Can you work these out from the model? Positions are in its coordinate system, mm. A direction names the side the tool comes from. Round coordinates to 2 decimals unless told otherwise and drop trailing zeros. Loops run counter-clockwise (first coordinate to the right, second up) from the corner with the lowest first, then second, coordinate; pieces in that order, holes last.
(1) Will these pins go through, and if not, where does the flat tip stop? pin 1 Ø3.5 at (x, z) = (-17, 1) entering from +Y; pin 2 Ø1 at (x, z) = (4, 1) entering from +Y; pin 3 Ø1.2 at (y, z) = (-2, 1) entering from +X; pin 4 Ø10 at (x, y) = (-12.5, 6.5) entering from -Z.
(2) I want a section at D-D on y = 21.5. Write out the boundary of the cut face in (x, z), plus the area to 3 significant figures.
(3) I want a section at B-B on z = -1. Write out the boundary of the cut face in (x, y), plus the area to 3 significant figures.
(4) If I drill on line 1 along X through (y, z) = (12, 0.25); line 2 along X through (y, z) = (-5.5, 2.75); line 3 along Y through (x, z) = (30, 3.5), over which ranges is the centre line in solid material (lowest first)?
(5) I want a section at C-C on y = 0.5. Write out the boundary of the cut face in (x, z).
(6) Thinking about a two-plate mould opening in Y: for faces 1 (the face through (-44, 0, -1)), 2 (the face through (0, -21.5, -1)), 3 (the face through (1, -30, -1)), which applies, released by +Y, released by -Y, zero draft, split by the parting line, or undercut?
(7) I want a section at A-A on x = 23. Write out the boundary of the cut face in (y, z).
(8) Which directions (+Z, -Z, +X, -X, +Y, -Y) give clear straight access to the entire face, cutting with the end or side of a thin tool? Please do faces 4 (the face through (20, -12.5, 1)), 5 (the face through (-1, -22.5, 2)), 6 (the face through (14, 16, 1)).
from build123d import *

# Parameters (mm, degrees)
SKETCH5_W           = 85
SKETCH5_H           = 45
SKETCH5_W_2         = 72
SKETCH5_H_2         = 25
BOSS_EXTRUDE3_DEPTH = 4
SKETCH10_W          = 88
SKETCH10_H          = 60
SKETCH10_W_2        = 72
SKETCH10_H_2        = 25
BOSS_EXTRUDE4_DEPTH = 3
SKETCH12_W          = 4
SKETCH12_H          = 15
CUT_EXTRUDE6_DEPTH  = 3
SKETCH13_W          = 43
SKETCH13_H          = 6
CUT_EXTRUDE7_DEPTH  = 3
SKETCH18_W          = 6.2
SKETCH18_H          = 5
CUT_EXTRUDE10_DEPTH = 9
SKETCH19_W          = 6.2
SKETCH19_H          = 0.5
CUT_EXTRUDE11_DEPTH = 10


with BuildPart() as part:
    # Sketch5 → Boss-Extrude3 (new body)
    with BuildSketch(Plane.XY):
        Rectangle(SKETCH5_W, SKETCH5_H)
        Rectangle(SKETCH5_W_2, SKETCH5_H_2, mode=Mode.SUBTRACT)
    extrude(amount=BOSS_EXTRUDE3_DEPTH)

    # Sketch10 → Boss-Extrude4 (add)
    with BuildSketch(Plane(origin=(0, 0, 0), x_dir=(-1, 0, 0), z_dir=(0, 0, -1))):
        Rectangle(SKETCH10_W, SKETCH10_H)
        Rectangle(SKETCH10_W_2, SKETCH10_H_2, mode=Mode.SUBTRACT)
    extrude(amount=BOSS_EXTRUDE4_DEPTH)

    # Sketch12 → Cut-Extrude6 (cut)
    with BuildSketch(Plane.XY.offset(4)):
        with Locations((-38, -0.264516135)):
            Rectangle(SKETCH12_W, SKETCH12_H)
    extrude(amount=-CUT_EXTRUDE6_DEPTH, mode=Mode.SUBTRACT)

    # Sketch13 → Cut-Extrude7 (cut)
    with BuildSketch(Plane.XY.offset(4)):
        with Locations((14.5, 15.5)):
            Rectangle(SKETCH13_W, SKETCH13_H)
    extrude(amount=-CUT_EXTRUDE7_DEPTH, mode=Mode.SUBTRACT)

    # Sketch18 → Cut-Extrude10 (cut)
    with BuildSketch(Plane(origin=(0, -12.5, 0), x_dir=(1, 0, 0), z_dir=(0, 1, 0))):
        with Locations((0, 0.5)):
            Rectangle(SKETCH18_W, SKETCH18_H)
    extrude(amount=-CUT_EXTRUDE10_DEPTH, mode=Mode.SUBTRACT)

    # Sketch19 → Cut-Extrude11 (cut)
    with BuildSketch(Plane(origin=(0, 0, 2), x_dir=(-1, 0, 0), z_dir=(0, 0, -1))):
        with Locations((0, -12.75)):
            Rectangle(SKETCH19_W, SKETCH19_H)
    extrude(amount=-CUT_EXTRUDE11_DEPTH, mode=Mode.SUBTRACT)


solid = part.part
Filled sheet:
1. pin 1: stops at y = 30
1. pin 2: stops at y = 22.5
1. pin 3: stops at x = 42.5
1. pin 4: passes through
2. outline: (-44, -3) - (44, -3) - (44, 0) - (42.5, 0) - (42.5, 4) - (-42.5, 4) - (-42.5, 0) - (-44, 0) - close
2. area: 604 mm2
3. outline: (-44, -30) - (44, -30) - (44, 30) - (-44, 30) - close; hole (-36, -12.5) - (-3.1, -12.5) - (-3.1, -21.5) - (3.1, -21.5) - (3.1, -12.5) - (36, -12.5) - (36, 12.5) - (-36, 12.5) - close
3. area: 3,420 mm2
4. line 1: x = -42.5 to -36, 36 to 42.5
4. line 2: x = -42.5 to -40, 36 to 42.5
4. line 3: y = -22.5 to -12.5, 18.5 to 22.5
5. outline: (-44, -3) - (-36, -3) - (-36, 1) - (-40, 1) - (-40, 4) - (-42.5, 4) - (-42.5, 0) - (-44, 0) - close; (36, -3) - (44, -3) - (44, 0) - (42.5, 0) - (42.5, 4) - (36, 4) - close
6. face 1: zero draft
6. face 2: undercut
6. face 3: released by -Y
7. outline: (-30, -3) - (-12.5, -3) - (-12.5, 4) - (-22.5, 4) - (-22.5, 0) - (-30, 0) - close; (12.5, -3) - (30, -3) - (30, 0) - (22.5, 0) - (22.5, 4) - (18.5, 4) - (18.5, 1) - (12.5, 1) - close
8. face 4: +Z, -Z
8. face 5: +Z, +X, -X, -Y
8. face 6: +Z
